Here's the drawing with two shaded views (mm, measured from the low corner). I have some questions. A direction names the side the tool comes from. Give positions to 0.01 mm unless a question says otherwise; leave off trailing zeros. Write each loop counter-clockwise with the first axis right and the second up, starting at its lowest first coordinate (ties: lowest second). Pieces come first, ordered by that corner, then holes. Notation, with made-up numbers: (83.5, 47) -> (104.5, 47) arc R15 ccw to (104.5, 76) -> close; hole circle Ø11 at (70.5, 16.25). An arc over 180 degrees is marked (long way). One line per question, with ' | ' between items.
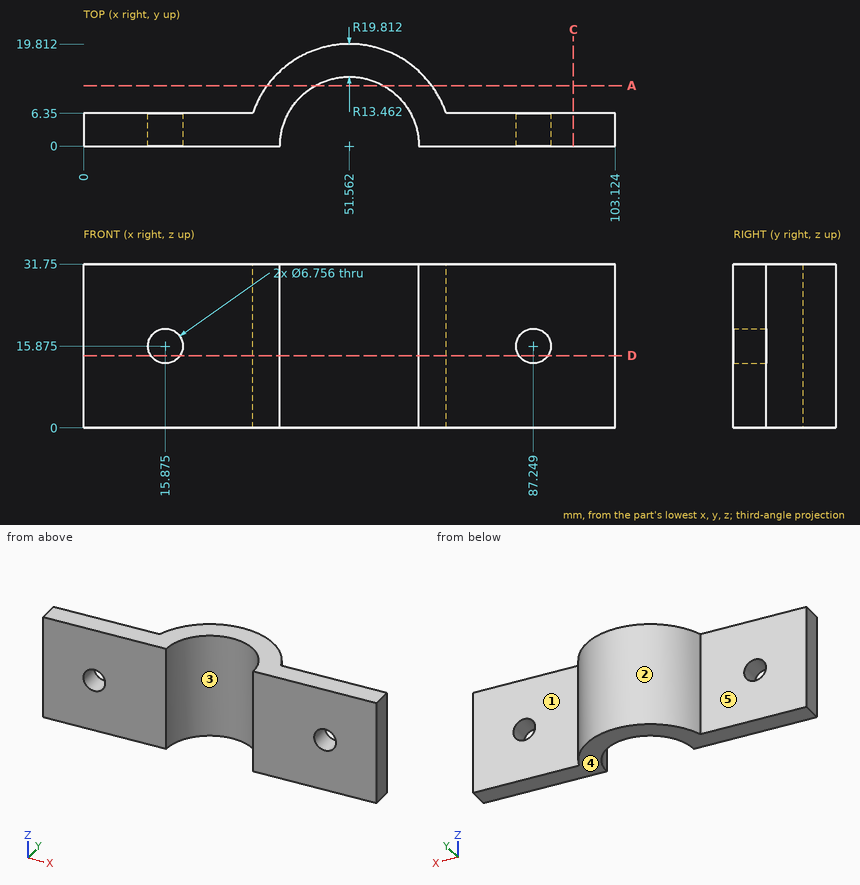
Q1. If I drill on line 1 along Z through (x, y) = (87, 2.5); line 2 along Y through (x, z) = (84.5, 23); line 3 along Z through (x, y) = (13, 4.25), over which ranges is the centre line in solid material (lowest first)?
Answer below:
line 1: z = 0 to 12.51, 19.24 to 31.75 | line 2: y = 0 to 6.35 | line 3: z = 0 to 14.1, 17.65 to 31.75
Q2. Imagine slicing it at C-C on x = 95. Please give me the cut outline in (y, z).
Answer below:
outline: (0, 0) -> (6.35, 0) -> (6.35, 31.75) -> (0, 31.75) -> close
Q3. Imagine slicing it at A-A on y = 11.75. Please give me the cut outline in (x, z), and give its area (3 significant figures).
Answer below:
outline: (35.61, 0) -> (44.99, 0) -> (44.99, 31.75) -> (35.61, 31.75) -> close; (58.13, 0) -> (67.51, 0) -> (67.51, 31.75) -> (58.13, 31.75) -> close | area: 596 mm^2
Q4. If we mould it in two halves opening along X, with no side actions, what happens to the marked faces 1, 2 and 3? For each: +X half, -X half, draft (parallel to the pull), parting line (faces both ways), or undercut.
Answer below:
face 1: draft | face 2: parting line | face 3: undercut
Q5. Will these pins go through, and if not, where does the flat tip stop? pin 1 (5 mm diameter, centred on x = 23.5, z = 8, fed in from +Y); pin 2 (3 mm diameter, centred on y = 13.5, z = 6, fed in from -X); pin 3 (2 mm diameter, centred on y = 6, z = 20.5, fed in from -X); pin 4 (8 mm diameter, centred on x = 50, z = 24, fed in from -Y).
Answer below:
pin 1: stops at y = 6.35 | pin 2: stops at x = 35.8 | pin 3: stops at x = 0 | pin 4: stops at y = 12.26
Q6. Imagine slicing it at D-D on z = 14. Count the separate pieces of the cut face and the enclosed holes in it, and give its area (3 significant figures).
Answer below:
separate pieces: 3 | enclosed holes: 0 | area: 668 mm^2
Q7. On a 3-axis mill with a long thin cutter (end or side, diameter ignored), from which of +Z, -Z, +X, -X, +Y, -Y can I reach the whole of each face in a straight line? I mean the marked faces 4 and 5. Say none if no direction works.
Answer below:
face 4: -Z, +X, -X, +Y, -Y | face 5: +Z, -Z, -X, +Y
